```python
from build123d import *

# Parameters (mm, degrees)
SKETCH1_W            = 60
SKETCH1_H            = 75
BOSS_EXTRUDE1_DEPTH  = 3
SKETCH2_W            = 60
SKETCH2_H            = 3
BOSS_EXTRUDE2_DEPTH  = 17
CUT_EXTRUDE1_REACH   = 52.944
SKETCH3_W            = 50
SKETCH3_H            = 33
CUT_EXTRUDE2_REACH   = 52.944
SKETCH4_R            = 2.45
M5_CLEARANCE_HOLE1_D = 5.5


with BuildPart() as part:
    # Sketch1 → Boss-Extrude1 (new body)
    with BuildSketch(Plane(origin=(0, 0, 0), x_dir=(1, 0, 0), z_dir=(0, 1, 0))):
        Rectangle(SKETCH1_W, SKETCH1_H)
    extrude(amount=BOSS_EXTRUDE1_DEPTH)

    # Sketch2 → Boss-Extrude2 (add)
    with BuildSketch(Plane(origin=(0, 3, 0), x_dir=(1, 0, 0), z_dir=(0, 1, 0))):
        with Locations((0, 36)):
            Rectangle(SKETCH2_W, SKETCH2_H)
    extrude(amount=BOSS_EXTRUDE2_DEPTH)

    # Sketch3 → Cut-Extrude1 (cut, up to next)
    with BuildSketch(Plane(origin=(0, 3, 0), x_dir=(1, 0, 0), z_dir=(0, 1, 0)), mode=Mode.PRIVATE) as cut_extrude1_sk1:
        with Locations((0, 5)):
            Rectangle(SKETCH3_W, SKETCH3_H)
    cut_extrude1_tool1 = extrude(cut_extrude1_sk1.sketch, amount=-CUT_EXTRUDE1_REACH, mode=Mode.PRIVATE) & part.part
    add(cut_extrude1_tool1.solids().sort_by_distance((0, 3, -5))[0], mode=Mode.SUBTRACT)

    # Sketch4 → Cut-Extrude2 (cut, up to next)
    with BuildSketch(Plane(origin=(0, 3, 0), x_dir=(1, 0, 0), z_dir=(0, 1, 0)), mode=Mode.PRIVATE) as cut_extrude2_sk1:
        with Locations(Location((-20, 25, 0), (0, 0, 270))):
            Circle(SKETCH4_R)
    cut_extrude2_tool1 = extrude(cut_extrude2_sk1.sketch, amount=-CUT_EXTRUDE2_REACH, mode=Mode.PRIVATE) & part.part
    # Sketch4 → Cut-Extrude2 (cut, up to next)
    with BuildSketch(Plane(origin=(0, 3, 0), x_dir=(1, 0, 0), z_dir=(0, 1, 0)), mode=Mode.PRIVATE) as cut_extrude2_sk2:
        with Locations(Location((20, 25, 0), (0, 0, 270))):
            Circle(SKETCH4_R)
    cut_extrude2_tool2 = extrude(cut_extrude2_sk2.sketch, amount=-CUT_EXTRUDE2_REACH, mode=Mode.PRIVATE) & part.part
    # Sketch4 → Cut-Extrude2 (cut, up to next)
    with BuildSketch(Plane(origin=(0, 3, 0), x_dir=(1, 0, 0), z_dir=(0, 1, 0)), mode=Mode.PRIVATE) as cut_extrude2_sk3:
        with Locations(Location((20, -15, 0), (0, 0, 270))):
            Circle(SKETCH4_R)
    cut_extrude2_tool3 = extrude(cut_extrude2_sk3.sketch, amount=-CUT_EXTRUDE2_REACH, mode=Mode.PRIVATE) & part.part
    # Sketch4 → Cut-Extrude2 (cut, up to next)
    with BuildSketch(Plane(origin=(0, 3, 0), x_dir=(1, 0, 0), z_dir=(0, 1, 0)), mode=Mode.PRIVATE) as cut_extrude2_sk4:
        with Locations(Location((-20, -15, 0), (0, 0, 270))):
            Circle(SKETCH4_R)
    cut_extrude2_tool4 = extrude(cut_extrude2_sk4.sketch, amount=-CUT_EXTRUDE2_REACH, mode=Mode.PRIVATE) & part.part
    add(cut_extrude2_tool1.solids().sort_by_distance((-20, 3, -25))[0], mode=Mode.SUBTRACT)
    add(cut_extrude2_tool2.solids().sort_by_distance((20, 3, -25))[0], mode=Mode.SUBTRACT)
    add(cut_extrude2_tool3.solids().sort_by_distance((20, 3, 15))[0], mode=Mode.SUBTRACT)
    add(cut_extrude2_tool4.solids().sort_by_distance((-20, 3, 15))[0], mode=Mode.SUBTRACT)

    # M5 Clearance Hole1 (through all)
    with Locations(Plane(origin=(22.5, 10, -37.5), x_dir=(-1, 0, 0), z_dir=(0, 0, -1))):
        with Locations((0, 0), (45, 0)):
            Hole(M5_CLEARANCE_HOLE1_D / 2)


solid = part.part
```
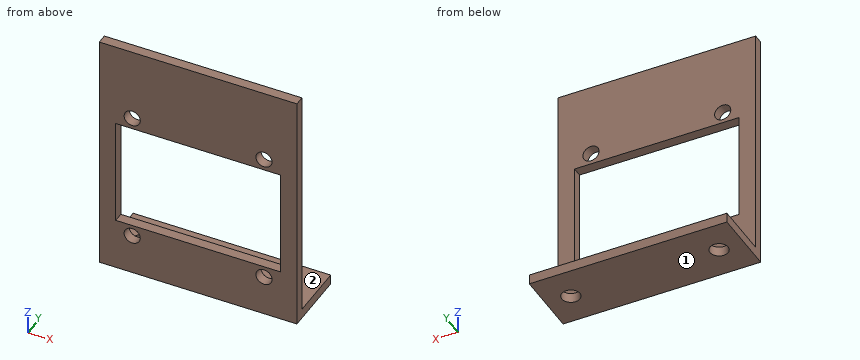
Here's how the part is built. I have some questions about the finished solid (model axes, mm). Face numbers are marked on the shaded views. A direction names the side the tool comes from. Round coordinates to 2 decimals unless told otherwise and drop trailing zeros. Loops run counter-clockwise (first coordinate to the right, second up) from the corner with the lowest first, then second, coordinate; pieces in that order, holes last.
1. If I drill on probe 1 along X at (y, z) = (0.8, -25); probe 2 along Z at (x, y) = (7.5, 2.5); probe 3 along Y at (x, z) = (-4, -29), over which ranges is the centre line in solid material (lowest first)?
Answers:
probe 1: x = -30 to -22.45, -17.55 to 17.55, 22.45 to 30
probe 2: z = -37.5 to -21.5, 11.5 to 37.5
probe 3: y = 0 to 3
2. Suppose I cut it at A-A, the plane y = 10. Please give me the cut outline in (x, z).
Answers:
outline: (-30, -37.5) - (-25.25, -37.5) - (-25.25, -34.5) - (-30, -34.5) - close; (-19.75, -37.5) - (19.75, -37.5) - (19.75, -34.5) - (-19.75, -34.5) - close; (25.25, -37.5) - (30, -37.5) - (30, -34.5) - (25.25, -34.5) - close
3. Suppose I cut it at C-C, the plane x = 5. Please give me the cut outline in (y, z).
Answers:
outline: (0, -37.5) - (20, -37.5) - (20, -34.5) - (3, -34.5) - (3, -21.5) - (0, -21.5) - close; (0, 11.5) - (3, 11.5) - (3, 37.5) - (0, 37.5) - close
4. Suppose I cut it at D-D, the plane z = -19. Please give me the cut outline in (x, y), and give its area (3 significant figures).
Answers:
outline: (-30, 0) - (-25, 0) - (-25, 3) - (-30, 3) - close; (25, 0) - (30, 0) - (30, 3) - (25, 3) - close
area: 30.0 mm2
5. Will these pins go through, and if not, where does the flat tip stop? pin 1 (5.5 mm diameter, centred on x = 20, z = -25, fed in from +Y); pin 2 (4 mm diameter, centred on x = -20, z = 15, fed in from +Y).
Answers:
pin 1: stops at y = 3
pin 2: passes through
6. Suppose I cut it at B-B, the plane z = 15. Please give me the cut outline in (x, y).
Answers:
outline: (-30, 0) - (-22.45, 0) - (-22.45, 3) - (-30, 3) - close; (-17.55, 0) - (17.55, 0) - (17.55, 3) - (-17.55, 3) - close; (22.45, 0) - (30, 0) - (30, 3) - (22.45, 3) - close
7. For the marked faces 1 and 2, which set-ups out of +Z, -Z, +X, -X, +Y, -Y let a thin tool reach every point of the face, with its end or its side?
Answers:
face 1: -Z, +X, -X, +Y, -Y
face 2: +Z, +X, -X, +Y
